```python
from build123d import *

# Parameters (mm, degrees)
F0_W           = 8
F0_H           = 5
F0_W_2         = 3
F0_W_3         = 5
F0_H_2         = 10
F0_H_3         = 20
F1_DEPTH       = 3
F2_DEPTH       = 19
F4_D           = 4.2
F4_CSINK_D     = 8
F4_CSINK_ANGLE = 90
F5_R           = 4


with BuildPart() as f1:
    # F0 (on Top) → F1 (new body)
    with BuildSketch(Plane.XY):
        Polygon((57.569327, 2.988489), (-19.430673, 2.988489), (-19.430673, -5.011511), (-14.430673, -5.011511), (-14.430673, -25.011511), (-19.430673, -25.011511), (-19.430673, -67.011511), (-14.430673, -67.011511), (-14.430673, -77.011511), (-11.430673, -77.011511), (-11.430673, -82.011511), (2.569327, -82.011511), (2.569327, -77.011511), (10.569327, -77.011511), (10.569327, -82.011511), (44.569327, -82.011511), (44.569327, -77.011511), (52.569327, -77.011511), (52.569327, -67.011511), (57.569327, -67.011511), (57.569327, -25.011511), (52.569327, -25.011511), (52.569327, -5.011511), (57.569327, -5.011511), align=None)
        with Locations((6.569327, -79.511511)):
            Rectangle(F0_W, F0_H)
        Polygon((-14.430673, -67.011511), (-19.430673, -67.011511), (-19.430673, -82.011511), (-14.430673, -82.011511), (-14.430673, -77.011511), align=None)
        with Locations((-12.930673, -79.511511)):
            Rectangle(F0_W_2, F0_H)
        Polygon((57.569327, -82.011511), (57.569327, -77.011511), (52.569327, -77.011511), (44.569327, -77.011511), (44.569327, -82.011511), align=None)
        with Locations((55.069327, -72.011511)):
            Rectangle(F0_W_3, F0_H_2)
        with Locations((55.069327, -15.011511)):
            Rectangle(F0_W_3, F0_H_3)
        with Locations((-16.930673, -15.011511)):
            Rectangle(F0_W_3, F0_H_3)
    extrude(amount=F1_DEPTH)

    # F0 (on Top) → F2 (join)
    with BuildSketch(Plane.XY):
        with Locations((-16.930673, -15.011511)):
            Rectangle(F0_W_3, F0_H_3)
        with Locations((55.069327, -15.011511)):
            Rectangle(F0_W_3, F0_H_3)
        with Locations((55.069327, -72.011511)):
            Rectangle(F0_W_3, F0_H_2)
        Polygon((57.569327, -82.011511), (57.569327, -77.011511), (52.569327, -77.011511), (44.569327, -77.011511), (44.569327, -82.011511), align=None)
        with Locations((6.569327, -79.511511)):
            Rectangle(F0_W, F0_H)
        Polygon((-14.430673, -67.011511), (-19.430673, -67.011511), (-19.430673, -82.011511), (-14.430673, -82.011511), (-14.430673, -77.011511), align=None)
        with Locations((-12.930673, -79.511511)):
            Rectangle(F0_W_2, F0_H)
    extrude(amount=F2_DEPTH)

    # F4 (through all)
    with Locations(Plane.XY.offset(3)):
        with Locations((6.069327, -11.011511), (32.069327, -11.011511), (6.069327, -63.011511), (32.069327, -63.011511), (32.069327, -37.011511), (6.069327, -37.011511)):
            CounterSinkHole(F4_D / 2, F4_CSINK_D / 2, counter_sink_angle=F4_CSINK_ANGLE)

    # F5
    f5_edges = [f1.edges().sort_by_distance(p)[0] for p in [
        (-16.930673, -25.011511, 3),
        (-16.930673, -67.011511, 3),
        (-11.430673, -79.511511, 3),
        (10.569327, -79.511511, 3),
        (2.569327, -79.511511, 3),
        (44.569327, -79.511511, 3),
        (55.069327, -25.011511, 3),
        (55.069327, -67.011511, 3),
        (55.069327, -5.011511, 3),
        (-16.930673, -5.011511, 3),
        (-14.430673, -15.011511, 3),
        (52.569327, -15.011511, 3),
    ]]
    fillet(f5_edges, radius=F5_R)


solid = f1.part
```
The model under review builds one solid part; all positions refer to its coordinate system, in mm. A direction names the side the tool comes from. Give positions to 0.01 mm unless a question says otherwise; leave off trailing zeros. Loops run counter-clockwise (first coordinate to the right, second up) from the corner with the lowest first, then second, coordinate; pieces in that order, holes last. Notation, with made-up numbers: (76.25, 6.25) - (126.25, 6.25) arc R31 ccw to (126.25, 39.25) - close; hole circle Ø8 at (67, 77.5). An arc over 180 degrees is marked (long way). Answer as a JSON object with one key per item and string values.
Q1. To check wall thickness, follow line 1 along X through (y, z) = (-78, 17.75); line 2 along X through (y, z) = (-18, 15.25); line 3 along Z through (x, y) = (7, -68). State the ranges of each line that lie inside material, in increasing order.
Worked out:
{"line 1": "x = -19.43 to -11.43, 2.57 to 10.57, 44.57 to 57.57", "line 2": "x = -19.43 to -14.43, 52.57 to 57.57", "line 3": "z = 0 to 3"}
Q2. Add section B-B on y = -16. State the section outline as (x, z) points, plus the area to 3 significant figures.
Worked out:
{"outline": "(-19.43, 0) - (57.57, 0) - (57.57, 19) - (52.57, 19) - (52.57, 7) arc R4 cw to (48.57, 3) - (-10.43, 3) arc R4 cw to (-14.43, 7) - (-14.43, 19) - (-19.43, 19) - close", "area": "398 mm^2"}
Q3. Add section D-D on z = 4.75. State the section outline as (x, y) points, plus the area to 3 significant figures.
Worked out:
{"outline": "(-19.43, -82.01) - (-10.74, -82.01) - (-10.74, -77.01) - (-14.43, -77.01) - (-14.43, -66.32) - (-19.43, -66.32) - close; (-19.43, -25.7) - (-13.74, -25.7) - (-13.74, -4.32) - (-19.43, -4.32) - close; (1.88, -82.01) - (11.26, -82.01) - (11.26, -77.01) - (1.88, -77.01) - close; (43.88, -82.01) - (57.57, -82.01) - (57.57, -66.32) - (52.57, -66.32) - (52.57, -77.01) - (43.88, -77.01) - close; (51.88, -25.7) - (57.57, -25.7) - (57.57, -4.32) - (51.88, -4.32) - close", "area": "509 mm^2"}
Q4. Add section A-A on z = 14.25. State the section outline as (x, y) points.
Worked out:
{"outline": "(-19.43, -82.01) - (-11.43, -82.01) - (-11.43, -77.01) - (-14.43, -77.01) - (-14.43, -67.01) - (-19.43, -67.01) - close; (-19.43, -25.01) - (-14.43, -25.01) - (-14.43, -5.01) - (-19.43, -5.01) - close; (2.57, -82.01) - (10.57, -82.01) - (10.57, -77.01) - (2.57, -77.01) - close; (44.57, -82.01) - (57.57, -82.01) - (57.57, -67.01) - (52.57, -67.01) - (52.57, -77.01) - (44.57, -77.01) - close; (52.57, -25.01) - (57.57, -25.01) - (57.57, -5.01) - (52.57, -5.01) - close"}
Q5. Mouldability with a two-part tool opening along X and no side actions: class faces 5 (the flat face through (20, 2.988, 1)), 6 (the flat face through (-14.431, -72, 11)) as +X half, -X half, draft (parallel to the pull), parting line (faces both ways), or undercut.
Worked out:
{"face 5": "draft", "face 6": "undercut"}
Q6. For faces 1 (the cylindrical face through (-16.9, -65.87, 4.2)), 2 (the flat face through (-17, -5.012, 13)), 3 (the cylindrical face through (11.71, -79.55, 4.2)), 4 (the flat face through (52.569, -15, 13)), list the 3-axis set-ups (+Z, -Z, +X, -X, +Y, -Y) from which the entire face can be reached by the end or side of a thin tool; tool diameter is ignored.
Worked out:
{"face 1": "+Z, +X, -X", "face 2": "+Z, +X, -X, +Y", "face 3": "+Z, +Y, -Y", "face 4": "+Z, +Y"}
Q7. Add section C-C on x = -13. State the section outline as (y, z) points.
Worked out:
{"outline": "(-82.01, 0) - (2.99, 0) - (2.99, 3) - (-1.01, 3) arc R4 cw to (-3.58, 3.93) - (-26.44, 3.93) arc R4 cw to (-29.01, 3) - (-77.01, 3) - (-77.01, 19) - (-82.01, 19) - close"}
Q8. Insertion check: pin 1 (4 mm diameter, centred on x = 6.07, y = -63.01, fed in from +Z); pin 2 (5 mm diameter, centred on x = 46.5, y = -69.5, fed in from +Z); pin 3 (2 mm diameter, centred on x = 46, z = 8.5, fed in from +Y); pin 4 (4 mm diameter, centred on x = 56, z = 15, fed in from +Y). Each pin has a flat end and moves straight along its axis. Give the tip position at first contact, or say it passes through.
Worked out:
{"pin 1": "passes through", "pin 2": "stops at z = 3", "pin 3": "stops at y = -77.01", "pin 4": "stops at y = -5.01"}
